```python
from build123d import *

# Parameters (mm, degrees)
BOSS_EXTRU_1_DEPTH      = 10
ESQUISSE2_R             = 2
ENL_V_MAT_EXTRU_1_DEPTH = 10
ESQUISSE4_W             = 4.610591942
ESQUISSE4_H             = 10
BOSS_EXTRU_3_DEPTH      = 6
ESQUISSE3_W             = 50
ESQUISSE3_H             = 20
BOSS_EXTRU_2_DEPTH      = 3


with BuildPart() as part:
    # Esquisse1 → Boss.-Extru.1 (new body)
    with BuildSketch(Plane.XY):
        with BuildLine():
            Line((-11, -4.795831523), (-5, -19.795831523))
            Line((-5, -19.795831523), (5, -19.795831523))
            Line((5, -19.795831523), (11, -4.795831523))
            ThreePointArc((11, -4.795831523), (0, 12), (-11, -4.795831523))
        make_face()
    extrude(amount=BOSS_EXTRU_1_DEPTH)

    # Esquisse2 → Enlèv. mat.-Extru.1 (cut)
    with BuildSketch(Plane(origin=(0, 0, 0), x_dir=(-1, 0, 0), z_dir=(0, 0, -1))):
        with Locations((0, -13)):
            Circle(ESQUISSE2_R)
    extrude(amount=-ENL_V_MAT_EXTRU_1_DEPTH, mode=Mode.SUBTRACT)

    # Esquisse4 → Boss.-Extru.3 (add)
    with BuildSketch(Plane(origin=(0, -19.795831523, 0), x_dir=(-1, 0, 0), z_dir=(0, -1, 0))):
        with Locations((0, -5)):
            Rectangle(ESQUISSE4_W, ESQUISSE4_H)
    extrude(amount=BOSS_EXTRU_3_DEPTH)

    # Esquisse3 → Boss.-Extru.2 (add)
    with BuildSketch(Plane(origin=(0, 0, 0), x_dir=(-1, 0, 0), z_dir=(0, 0, -1))):
        Rectangle(ESQUISSE3_W, ESQUISSE3_H)
    extrude(amount=BOSS_EXTRU_2_DEPTH)


solid = part.part
```
Read the model definition and answer for the solid it produces. Units are mm, in the model's axes. A direction names the side the tool comes from. Give positions to 0.01 mm unless a question says otherwise; leave off trailing zeros. Order: outer loops, then holes, each group sorted by start corner. A loop starts at its lowest first (then second) coordinate and runs counter-clockwise, first axis right, second up. Notation, with made-up numbers: (-13.5, -36.75) -> (25.5, -36.75) arc R21 cw to (25.5, -26.75) -> close; hole circle Ø11 at (43, -31.5). An arc over 180 degrees is marked (long way). One line per item, written item: value. Start each with the question number.
(1) Straight lines are drawn through the part: L1, parallel to Y at x = 0, z = 6.75; L2, parallel to X at y = -14.5, z = 7.25; L3, parallel to Z at x = 20.5, y = 5. For each, find the intervals that lie inside material, in ascending order.
(2) For a pull along X with two mould halves and no side action, classify faces 1 (the flat face through (-8.042, -12.191, 4.93)), 2 (the cylindrical face through (0, -11, 5)), 3 (the flat face through (-4, -19.796, 5)), 4 (the flat face through (25, 0, -1)) as released by +X, released by -X, zero draft, split by the parting line, or undercut.
(3) The part is cut by section C-C (y = 0). Determine the outline of the cut face in (x, z), and give its area (3 significant figures).
(4) Flat-ended cylindrical pins translate along their axes: P1, Ø6.5, axis at y = -22.5, z = 4, coming from the -X side; P2, Ø4, axis at x = 7.5, z = 5, coming from the +Y side; P3, Ø1.5, axis at y = -11.5, z = 8, coming from the +X side. Find the tip coordinate at first contact, or state that the pin passes through.
(5) A tool of negligible diameter and unlimited length cuts with its end or side. For faces 5 (the flat face through (0, 10, -1)), 6 (the cylindrical face through (0, 12, 5)), 7 (the flat face through (4, -19.796, 5)), from which of +Z, -Z, +X, -X, +Y, -Y can it reach the whole face along a straight path? Write none if from no direction.
(6) The part is cut by section A-A (z = 8.5). Determine the outline of the cut face in (x, y).
(7) The part is cut by section D-D (y = -13). Determine the outline of the cut face in (x, z), and give its area (3 significant figures).
(8) The part is cut by section B-B (x = 0). Determine the outline of the cut face in (y, z).
Taken from the geometry:
1. L1: -25.8 to -15, -11 to 12
1. L2: -7.12 to -1.32, 1.32 to 7.12
1. L3: -3 to 0
2. face 1: released by -X
2. face 2: undercut
2. face 3: zero draft
2. face 4: released by +X
3. outline: (-25, -3) -> (25, -3) -> (25, 0) -> (12, 0) -> (12, 10) -> (-12, 10) -> (-12, 0) -> (-25, 0) -> close
3. area: 390 mm^2
4. P1: x = -5.22
4. P2: y = 10.67
4. P3: x = 8.62
5. face 5: -Z, +X, -X, +Y
5. face 6: +Z
5. face 7: +Z, -Z, +X, -Y
6. outline: (-11, -4.8) -> (-5, -19.8) -> (-2.31, -19.8) -> (-2.31, -25.8) -> (2.31, -25.8) -> (2.31, -19.8) -> (5, -19.8) -> (11, -4.8) arc R12 ccw (long way) to start; hole circle Ø4 at (0, -13)
7. outline: (-7.72, 0) -> (-2, 0) -> (-2, 10) -> (-7.72, 10) -> close; (2, 0) -> (7.72, 0) -> (7.72, 10) -> (2, 10) -> close
7. area: 114 mm^2
8. outline: (-25.8, 0) -> (-15, 0) -> (-15, 10) -> (-25.8, 10) -> close; (-11, 0) -> (-10, 0) -> (-10, -3) -> (10, -3) -> (10, 0) -> (12, 0) -> (12, 10) -> (-11, 10) -> close
